Could you check a few things on this model? Use its own coordinates, in mm. A direction names the side the tool comes from. Coordinates: 2 decimals unless noted, no trailing zeros. Loops run counter-clockwise (first coordinate to the right, second up) from the corner with the lowest first, then second, coordinate; pieces in that order, holes last.
from build123d import *

# Parameters (mm, degrees)
RESSALTO_EXTRUS_O1_START            = -4.5
RESSALTO_EXTRUS_O1_OUTLINE_R        = 2.5
RESSALTO_EXTRUS_O1_DEPTH            = 4.5
RESSALTO_EXTRUS_O1_START_2          = -3.5
RESSALTO_EXTRUS_O1_2_OUTLINE_R      = 2.695
RESSALTO_EXTRUS_O1_2_OUTLINE_R_2    = 2.5
RESSALTO_EXTRUS_O1_2_DEPTH          = 3.5
RESSALTO_EXTRUS_O1_3_OUTLINE_R      = 2.5
RESSALTO_EXTRUS_O1_3_DEPTH          = 0.5
ESBO_O2_R                           = 2.695
RESSALTO_EXTRUS_O2_DEPTH            = 3.5
FURO_ROSCADO_DE_M3X0_51_D           = 2.5
FURO_ROSCADO_DE_M3X0_51_CSINK_D     = 3.05
FURO_ROSCADO_DE_M3X0_51_CSINK_ANGLE = 90
CORTE_EXTRUS_O1_START               = -7.5
ESBO_O7_R                           = 2.695
ESBO_O7_R_2                         = 2.1
CORTE_EXTRUS_O1_DEPTH               = 7.5
ESBO_O8_R                           = 2.1
ESBO_O8_R_2                         = 1.6
CORTE_EXTRUS_O2_DEPTH               = 0.5


with BuildPart() as part:
    # Ressalto-extrusão1: read off the stored shape, not the designer's step
    # Ressalto-extrusão1 outline → Ressalto-extrusão1 (new body)
    with BuildSketch(Plane(origin=(0, 4.5, 0), x_dir=(1, 0, 0), z_dir=(0, 1, 0)).offset(RESSALTO_EXTRUS_O1_START)):
        Circle(RESSALTO_EXTRUS_O1_OUTLINE_R)
    extrude(amount=RESSALTO_EXTRUS_O1_DEPTH)

    # Ressalto-extrus_o1 2 outline → Ressalto-extrus_o1 2 (add)
    with BuildSketch(Plane(origin=(0, 4.5, 0), x_dir=(1, 0, 0), z_dir=(0, 1, 0)).offset(RESSALTO_EXTRUS_O1_START_2)):
        Circle(RESSALTO_EXTRUS_O1_2_OUTLINE_R)
        Circle(RESSALTO_EXTRUS_O1_2_OUTLINE_R_2, mode=Mode.SUBTRACT)
    extrude(amount=RESSALTO_EXTRUS_O1_2_DEPTH)

    # Ressalto-extrus_o1 3 outline → Ressalto-extrus_o1 3 (add)
    with BuildSketch(Plane(origin=(0, 4.5, 0), x_dir=(1, 0, 0), z_dir=(0, 1, 0)).offset(RESSALTO_EXTRUS_O1_START)):
        Polygon((0, 3.695041723), (-3.2, 1.847520861), (-3.2, -1.847520861), (0, -3.695041723), (3.2, -1.847520861), (3.2, 1.847520861), align=None)
        Circle(RESSALTO_EXTRUS_O1_3_OUTLINE_R, mode=Mode.SUBTRACT)
    extrude(amount=RESSALTO_EXTRUS_O1_3_DEPTH)

    # Esboço2 → Ressalto-extrusão2 (add)
    with BuildSketch(Plane(origin=(0, 4.5, 0), x_dir=(1, 0, 0), z_dir=(0, 1, 0))):
        with Locations(Location((0, 0, 0), (0, 0, 90))):
            Circle(ESBO_O2_R)
    extrude(amount=RESSALTO_EXTRUS_O2_DEPTH)

    # Furo roscado de M3x0.51 (through all)
    with Locations(Plane(origin=(0, 8, 0), x_dir=(1, 0, 0), z_dir=(0, 1, 0))):
        with Locations((0, 0)):
            CounterSinkHole(FURO_ROSCADO_DE_M3X0_51_D / 2, FURO_ROSCADO_DE_M3X0_51_CSINK_D / 2, counter_sink_angle=FURO_ROSCADO_DE_M3X0_51_CSINK_ANGLE)

    # Esboço7 → Corte-extrusão1 (cut)
    with BuildSketch(Plane(origin=(0, 8, 0), x_dir=(1, 0, 0), z_dir=(0, 1, 0)).offset(CORTE_EXTRUS_O1_START)):
        Circle(ESBO_O7_R)
        with Locations(Location((0, 0, 0), (0, 0, 270))):
            Circle(ESBO_O7_R_2, mode=Mode.SUBTRACT)
    extrude(amount=CORTE_EXTRUS_O1_DEPTH, mode=Mode.SUBTRACT)

    # Esboço8 → Corte-extrusão2 (cut)
    with BuildSketch(Plane(origin=(0, 0.5, 0), x_dir=(1, 0, 0), z_dir=(0, 1, 0))):
        with Locations(Location((0, 0, 0), (0, 0, 270))):
            Circle(ESBO_O8_R)
        with Locations(Location((0, 0, 0), (0, 0, 270))):
            Circle(ESBO_O8_R_2, mode=Mode.SUBTRACT)
    extrude(amount=CORTE_EXTRUS_O2_DEPTH, mode=Mode.SUBTRACT)


solid = part.part
(1) Imagine slicing it at A-A, the plane z = 0. Write out the boundary of the cut face in (x, y) (3 decimals).
Answers:
outline: (-3.2, 0) - (-1.25, 0) - (-1.25, 7.725) - (-1.525, 8) - (-2.1, 8) - (-2.1, 1) - (-1.6, 1) - (-1.6, 0.5) - (-3.2, 0.5) - close; (1.25, 0) - (3.2, 0) - (3.2, 0.5) - (1.6, 0.5) - (1.6, 1) - (2.1, 1) - (2.1, 8) - (1.525, 8) - (1.25, 7.725) - close
(2) For pin 1 (1 mm diameter, centred on y = 4.5, z = -1.5, fed in from +X); pin 2 (3 mm diameter, centred on x = 0, z = 0, fed in from +Y) (3 decimals); pin 3 (2 mm diameter, centred on x = -2, y = 5.5, fed in from +Z); pin 4 (1.3 mm diameter, centred on x = 1, z = 1, fed in from -Y), each with a flat end and sliding along its axis, tell me the tip position at first contact or that it passes through.
Answers:
pin 1: stops at x = 1.85
pin 2: stops at y = 7.975
pin 3: stops at z = 1.85
pin 4: stops at y = 0
(3) Imagine slicing it at B-B, the plane y = 3.75. Write out the boundary of the cut face in (x, z).
Answers:
outline: circle Ø4.2 at (0, 0); hole circle Ø2.5 at (0, 0)
(4) Imagine slicing it at D-D, the plane z = 2.25. Write out the boundary of the cut face in (x, y), and give its area (3 significant figures).
Answers:
outline: (-2.5, 0) - (2.5, 0) - (2.5, 0.5) - (-2.5, 0.5) - close
area: 2.50 mm2
(5) Imagine slicing it at C-C, the plane x = 2.5. Write out the boundary of the cut face in (y, z).
Answers:
outline: (0, -2.25) - (0.5, -2.25) - (0.5, 2.25) - (0, 2.25) - close
(6) Which directions (+Z, -Z, +X, -X, +Y, -Y) give clear straight access to the entire face, cutting with the end or side of a thin tool? Please do faces 4 (the face through (-0.97, 0.75, -1.27)), 5 (the face through (-1.578, 0.246, -2.784)), 6 (the face through (0.631, 4.451, 2.003)).
Answers:
face 4: none
face 5: -Z, -X, +Y, -Y
face 6: +Y
(7) I need wall thicknesses on probe 1 along Y at (x, z) = (-0.75, 1.5); probe 2 along Y at (x, z) = (-3, 0); probe 3 along Z at (x, y) = (0.25, 2.5). Which ranges of each line are inside material? Lowest first, please.
Answers:
probe 1: y = 0 to 0.5, 1 to 8
probe 2: y = 0 to 0.5
probe 3: z = -2.09 to -1.22, 1.22 to 2.09
(8) We'd pull the mould along Y, two halves only. Please class faces 1 (the face through (1, 0.5, 2)), 2 (the face through (-1.62, 0.25, 2.76)), 3 (the face through (0, 0, 2)): +Y half, -Y half, draft (parallel to the pull), parting line (faces both ways), or undercut.
Answers:
face 1: undercut
face 2: draft
face 3: -Y half
